from build123d import *

# Parameters (mm, degrees)
SKIZZE1_W                            = 49
SKIZZE1_H                            = 30
AUFSATZ_LINEAR_AUSTRAGEN1_DEPTH      = 1.5
SKIZZE2_W                            = 49
SKIZZE2_H                            = 20
AUFSATZ_LINEAR_AUSTRAGEN2_DEPTH      = 9
SKIZZE3_R                            = 1.8
SCHNITT_LINEAR_AUSTRAGEN1_DEPTH      = 10
SCHNITT_LINEAR_AUSTRAGEN1_DEPTH_BACK = 2.5
SKIZZE4_W                            = 42
SKIZZE4_H                            = 20.4
AUFSATZ_LINEAR_AUSTRAGEN3_DEPTH      = 3.5
SKIZZE5_W                            = 9.3
SKIZZE5_H                            = 10
SKIZZE5_W_2                          = 5.202111929
SKIZZE5_H_2                          = 5.340958118
SKIZZE5_W_3                          = 5.892281305
SKIZZE5_H_3                          = 9.90280044
SKIZZE5_H_4                          = 4.8
AUFSATZ_LINEAR_AUSTRAGEN4_DEPTH      = 4.2


with BuildPart() as part:
    # Skizze1 → Aufsatz-Linear austragen1 (new body)
    with BuildSketch(Plane(origin=(0, 0, 0), x_dir=(1, 0, 0), z_dir=(0, 1, 0))):
        with Locations((-24.5, -15)):
            Rectangle(SKIZZE1_W, SKIZZE1_H)
    extrude(amount=AUFSATZ_LINEAR_AUSTRAGEN1_DEPTH)

    # Skizze2 → Aufsatz-Linear austragen2 (add)
    with BuildSketch(Plane(origin=(0, 1.5, 0), x_dir=(1, 0, 0), z_dir=(0, 1, 0))):
        with Locations((-24.5, -10)):
            Rectangle(SKIZZE2_W, SKIZZE2_H)
    extrude(amount=AUFSATZ_LINEAR_AUSTRAGEN2_DEPTH)

    # Skizze3 → Schnitt-Linear austragen1 (cut, two sides)
    with BuildSketch(Plane(origin=(0, 1.5, 0), x_dir=(1, 0, 0), z_dir=(0, 1, 0))) as schnitt_linear_austragen1_sk:
        with Locations((-46.5, -27.5)):
            Circle(SKIZZE3_R)
    extrude(amount=SCHNITT_LINEAR_AUSTRAGEN1_DEPTH, mode=Mode.SUBTRACT)
    extrude(schnitt_linear_austragen1_sk.sketch, amount=-SCHNITT_LINEAR_AUSTRAGEN1_DEPTH_BACK, mode=Mode.SUBTRACT)

    # Spiegeln1: part across plane


with BuildPart() as part_1:
    add(part.part)
    add(part.part.mirror(Plane(origin=(0, 1.5, 0), x_dir=(0, 0, 1), z_dir=(-1, 0, 0))))

    # Spiegeln2: part across plane


with BuildPart() as part_2:
    add(part_1.part)
    add(part_1.part.mirror(Plane(origin=(0, 1.5, 0), x_dir=(1, 0, 0), z_dir=(0, 0, 1))))

    # Skizze4 → Aufsatz-Linear austragen3 (add)
    with BuildSketch(Plane.XZ):
        with Locations((-20, 19.8)):
            Rectangle(SKIZZE4_W, SKIZZE4_H)
    extrude(amount=AUFSATZ_LINEAR_AUSTRAGEN3_DEPTH)

    # Skizze5 → Aufsatz-Linear austragen4 (add)
    with BuildSketch(Plane.XZ.offset(3.5)):
        with Locations((-43.15, 19.8)):
            Rectangle(SKIZZE5_W, SKIZZE5_H)
        with Locations((-28.561234427, 15.050145035)):
            Rectangle(SKIZZE5_W_2, SKIZZE5_H_2)
        with Locations((-17.866219882, 19.8)):
            Rectangle(SKIZZE5_W_3, SKIZZE5_H_3)
        with Locations((3.15, 17.4)):
            Rectangle(SKIZZE5_W, SKIZZE5_H_4)
    extrude(amount=AUFSATZ_LINEAR_AUSTRAGEN4_DEPTH)


solid = part_2.part
Build history of the part. All positions in model axes, mm. A direction names the side the tool comes from. Round coordinates to 2 decimals unless told otherwise and drop trailing zeros. Write each loop counter-clockwise with the first axis right and the second up, starting at its lowest first coordinate (ties: lowest second). Pieces come first, ordered by that corner, then holes. Notation, with made-up numbers: M 54,-35.75 L 95,-35.75 A33 ccw 95,-4.75 Z; hole C 48.5,-6.5 d1. An arc over 180 degrees is marked long. Use CSV: the item, a comma, the result in double quotes.
1. Saw through at B-B (x = 46.5). Give the cut face in (y, z), plus the area to 3 significant figures.
Reply:
outline,"M 0,-30 L 1.5,-30 L 1.5,-29.3 L 0,-29.3 Z; M 0,-25.7 L 1.5,-25.7 L 1.5,-20 L 10.5,-20 L 10.5,20 L 1.5,20 L 1.5,25.7 L 0,25.7 Z; M 0,29.3 L 1.5,29.3 L 1.5,30 L 0,30 Z"
area,"439 mm²"
2. Saw through at A-A (z = -27.5). Give the cut face in (x, y), plus the area to 3 significant figures.
Reply:
outline,"M -49,0 L -48.3,0 L -48.3,1.5 L -49,1.5 Z; M -44.7,0 L 44.7,0 L 44.7,1.5 L -44.7,1.5 Z; M 48.3,0 L 49,0 L 49,1.5 L 48.3,1.5 Z"
area,"136 mm²"
3. Saw through at D-D (x = -46.5). Give the cut face in (y, z), plus the area to 3 significant figures.
Reply:
outline,"M -7.7,14.8 L -3.5,14.8 L -3.5,24.8 L -7.7,24.8 Z; M 0,-30 L 1.5,-30 L 1.5,-29.3 L 0,-29.3 Z; M 0,-25.7 L 1.5,-25.7 L 1.5,-20 L 10.5,-20 L 10.5,20 L 1.5,20 L 1.5,25.7 L 0,25.7 Z; M 0,29.3 L 1.5,29.3 L 1.5,30 L 0,30 Z"
area,"481 mm²"
4. Saw through at C-C (x = 5). Give the cut face in (y, z).
Reply:
outline,"M -7.7,15 L -3.5,15 L -3.5,19.8 L -7.7,19.8 Z; M 0,-30 L 1.5,-30 L 1.5,-20 L 10.5,-20 L 10.5,20 L 1.5,20 L 1.5,30 L 0,30 Z"
5. Flat gauge pins, fed straight in: pin 1 (2 mm diameter, centred on y = -5.5, z = 15, fed in from +X); pin 2 (7 mm diameter, centred on x = 23.5, y = 8, fed in from -Z); pin 3 (2 mm diameter, centred on x = -41.5, y = -4.5, fed in from +Z). Where does each tip first touch, or does it go through?
Reply:
pin 1,"stops at x = 7.8"
pin 2,"stops at z = -20"
pin 3,"stops at z = 24.8"
6. Two-plate mould, pull along Z, no slides. Class faces 1 (the face through (-45.532, 0.76, -25.982)), 2 (the face through (1, 6, -20)), 3 (the face through (-10, 0, 30)): +Z half, -Z half, draft (parallel to the pull), parting line (faces both ways), or undercut.
Reply:
face 1,"undercut"
face 2,"-Z half"
face 3,"+Z half"
7. Tool access for faces 4 (the face through (-25.96, -6, 15)), 5 (the face through (1, 1.5, 25)): list every direction of +Z, -Z, +X, -X, +Y, -Y with a clear straight run to the whole face (end or side of a thin tool).
Reply:
face 4,"+Z, -Z, -Y"
face 5,"+Z, +X, -X, +Y"
8. Wall check: probe 1 along Z at (x, y) = (-46.5, 0.35); probe 2 along X at (y, z) = (1, 27.5); probe 3 along Z at (x, y) = (15.5, 3). Give the ranges that are in metal, low to high. Write a range as from..to.
Reply:
probe 1,"z = -30..-29.3, -25.7..25.7, 29.3..30"
probe 2,"x = -49..-48.3, -44.7..44.7, 48.3..49"
probe 3,"z = -20..20"
